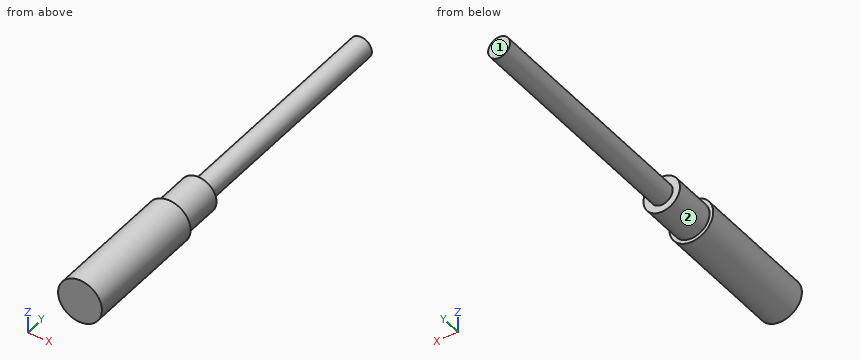
from build123d import *

# Parameters (mm, degrees)
F0_R     = 1.5
F1_DEPTH = 33
F2_R     = 2.5016426342
F2_R_2   = 1.5
F3_DEPTH = 6
F4_R     = 3
F4_R_2   = 2.5016426342
F5_DEPTH = 18


with BuildPart() as f1:
    # F0 (on Front) → F1 (new body)
    with BuildSketch(Plane.XZ):
        Circle(F0_R)
    extrude(amount=F1_DEPTH)

    # F2 (on face) → F3 (join)
    with BuildSketch(Plane.XZ.offset(33)):
        Circle(F2_R)
        Circle(F2_R_2, mode=Mode.SUBTRACT)
        Circle(F2_R_2)
    extrude(amount=F3_DEPTH)

    # F4 (on face) → F5 (join)
    with BuildSketch(Plane.XZ.offset(39)):
        Circle(F4_R)
        Circle(F4_R_2, mode=Mode.SUBTRACT)
        Circle(F4_R_2)
    extrude(amount=F5_DEPTH)


solid = f1.part
The listing builds one solid part. Answer for the finished solid, in the listing's coordinates (mm). Face numbers are marked on the shaded views. A direction names the side the tool comes from. Give positions to 0.01 mm unless a question says otherwise; leave off trailing zeros. Loops run counter-clockwise (first coordinate to the right, second up) from the corner with the lowest first, then second, coordinate; pieces in that order, holes last.
Item 1: A tool of negligible diameter and unlimited length cuts with its end or side. For the marked faces 1 and 2, from which of +Z, -Z, +X, -X, +Y, -Y can it reach the whole face along a straight path? Write none if from no direction.
Derived:
face 1: +Z, -Z, +X, -X, +Y
face 2: +Y
Item 2: A cutting plane is placed at C-C (y = -50). Give the vertices of the cut face in (x, z).
Derived:
outline: circle Ø6 at (0, 0)
Item 3: Each of these flat-tipped pins is pushed along its axis until it touches: pin 1 Ø2.5 at (x, z) = (-0.5, 1) entering from +Y; pin 2 Ø3 at (x, y) = (0.5, -26) entering from -Z; pin 3 Ø1 at (x, z) = (-2, 2) entering from +Y; pin 4 Ø3 at (x, y) = (-2, -30) entering from -Z. Where does it stop, or does it pass through?
Derived:
pin 1: stops at y = 0
pin 2: stops at z = -1.5
pin 3: stops at y = -33
pin 4: stops at z = -1.41
Item 4: A cutting plane is placed at B-B (x = 0). Give the vertices of the cut face in (y, z).
Derived:
outline: (-57, -3) - (-39, -3) - (-39, -2.5) - (-33, -2.5) - (-33, -1.5) - (0, -1.5) - (0, 1.5) - (-33, 1.5) - (-33, 2.5) - (-39, 2.5) - (-39, 3) - (-57, 3) - close
Item 5: A cutting plane is placed at A-A (z = 0). Give the vertices of the cut face in (x, y).
Derived:
outline: (-3, -57) - (3, -57) - (3, -39) - (2.5, -39) - (2.5, -33) - (1.5, -33) - (1.5, 0) - (-1.5, 0) - (-1.5, -33) - (-2.5, -33) - (-2.5, -39) - (-3, -39) - close
Item 6: A cutting plane is placed at D-D (y = -29). Give the vertices of the cut face in (x, z), then the cut area to 3 significant figures.
Derived:
outline: circle Ø3 at (0, 0)
area: 7.07 mm2
Item 7: Find the intervals of material crossed by line 1 along X through (y, z) = (-48.5, 0.25); line 2 along Y through (x, z) = (-1.9, 0.15); line 3 along Z through (x, y) = (-0.15, -32), in increasing order.
Derived:
line 1: x = -2.99 to 2.99
line 2: y = -57 to -33
line 3: z = -1.49 to 1.49
